Geometry check sheet. Reference: the model listing, model coordinates, mm. A direction names the side the tool comes from. Coordinates: 2 decimals unless noted, no trailing zeros. Order: outer loops, then holes, each group sorted by start corner. A loop starts at its lowest first (then second) coordinate and runs counter-clockwise, first axis right, second up. Notation, with made-up numbers: (26.25, 65) - (66.25, 65) arc R15 ccw to (66.25, 73) - close; hole circle Ø7 at (37.5, 6.25). An arc over 180 degrees is marked (long way). One line per item, written item: value. Start each with the question number.
Autodesk Inventor part; units mm, degrees
ref_plane "YZ Plane" through (0, 0, 0) normal (1, 0, 0) x (0, 1, 0)
ref_plane "XZ Plane" through (0, 0, 0) normal (0, 1, 0) x (-1, 0, 0)
ref_plane "XY Plane" through (0, 0, 0) normal (0, 0, 1) x (1, 0, 0)
sketch "Sketch1" plane through (0, 0, 0) normal (0, 0, 1) x (1, 0, 0)
  line L0 (-64, 10) -> (0, 10)
  line L1 (0, 10) -> (0, 0)
  line L2 (0, 0) -> (-64, 0)
  line L3 (-64, 0) -> (-64, 10)
  dimension "d0" = 64
  dimension "d1" = 10
extrude "Extrusion1" add sketch "Sketch1" along normal blind 50
sketch "Sketch2" plane through (0, 0, 50) normal (0, 0, 1) x (1, 0, 0)
  line L0 (0, 10) -> (-64, 10)
  line L1 (-64, 10) -> (-64, 0)
  line L2 (-64, 0) -> (0, 0)
  line L3 (0, 0) -> (0, 10)
  circle A0 centre (-57, 5) radius 2.5
  circle A1 centre (-7, 5) radius 2.5
  line L4 (-32, 17) -> (-32, -12)
  line L5 (-64, 10) -> (-64, 0)
  line L6 (-64, 5) -> (0, 5)
  dimension "d4" = 50
  dimension "d5" = 5
  dimension "d6" = 32
extrude "Extrusion2" cut sketch "Sketch2" against normal blind 18 contours L6 A1 | A1 L6 | L6 A0 | A0 L6
sketch "Sketch3" plane through (0, 0, 50) normal (0, 0, 1) x (1, 0, 0)
  circle A0 centre (-7, 5) radius 2.5
  circle A1 centre (-57, 5) radius 2.5
  line L0 (0, 10) -> (-64, 10)
  line L1 (-64, 10) -> (-64, 0)
  line L2 (-64, 0) -> (0, 0)
  line L3 (0, 0) -> (0, 10)
  line L4 (-64, 0) -> (0, 0)
  line L5 (-50, 10) -> (-14, 10)
  line L6 (-14, 10) -> (-14, 0)
  line L7 (-14, 0) -> (-50, 0)
  line L8 (-50, 0) -> (-50, 10)
  dimension "d9" = 14
  dimension "d10" = 14
ref_plane "Work Plane1" through (-32, 0, 0) normal (-1, 0, 0) x (0, 0, 1)
extrude "Extrusion3" cut sketch "Sketch3" against normal blind 15 contours L6 L2 L8 L0
sketch "Sketch4" plane through (-64, 0, 0) normal (0, -1, 0) x (1, 0, 0)
  line L0 (14, 35) -> (14, 50)
  line L1 (0, 50) -> (14, 50)
  line L2 (0, 0) -> (0, 50)
  line L3 (64, 0) -> (0, 0)
  line L4 (64, 0) -> (64, 50)
  line L5 (50, 50) -> (64, 50)
  line L6 (50, 50) -> (50, 35)
  line L7 (50, 35) -> (14, 35)
  line L8 (9.5, 50) -> (9.5, 32)
  line L9 (4.5, 50) -> (4.5, 32)
sketch "Sketch5" plane through (-64, 0, 0) normal (0, -1, 0) x (1, 0, 0)
  line L0 (4, 45) -> (10, 45)
  line L1 (10, 45) -> (10, 42)
  line L2 (10, 42) -> (4, 42)
  line L3 (4, 42) -> (4, 45)
  line L4 (4.5, 50) -> (9.5, 50)
  line L5 (7, 50) -> (7, 38)
  line L6 (0, 50) -> (14, 50)
  point P0 (64, 0)
  point P1 (7, 50)
  dimension "d13" = 6
  dimension "d14" = 3
  dimension "d15" = 5
extrude "Extrusion4" cut sketch "Sketch5" against normal blind 8.5
mirror "Mirror1" about plane through (-32, 0, 0) normal (-1, 0, 0) of "Extrusion4"
sketch "Sketch6" plane through (0, 0, 0) normal (0, 0, -1) x (-1, 0, 0)
  line L0 (64, 10) -> (0, 10)
  line L1 (0, 10) -> (0, 0)
  line L2 (0, 0) -> (64, 0)
  line L3 (64, 0) -> (64, 10)
  line L4 (0, 0) -> (64, 0)
  line L5 (64, 0) -> (64, -15)
  line L6 (64, -15) -> (0, -15)
  line L7 (0, -15) -> (0, 0)
  dimension "d30" = 15
extrude "Extrusion5" add sketch "Sketch6" against normal blind 4 contours L5 L6 L7 L2
sketch "Sketch7" plane through (0, 0, 4) normal (0, 0, 1) x (1, 0, 0)
  line L0 (0, -15) -> (0, 0)
  line L1 (-64, 0) -> (0, 0)
  line L2 (-64, 0) -> (-64, -15)
  line L3 (-64, -15) -> (0, -15)
  line L4 (-54, -7) -> (-10, -7) construction
  line L5 (-54, -9.5) -> (-10, -9.5)
  line L6 (-10, -4.5) -> (-54, -4.5)
  arc A0 (-54, -4.5) -> (-54, -9.5) centre (-54, -7) ccw
  arc A1 (-10, -9.5) -> (-10, -4.5) centre (-10, -7) ccw
  point P0 (-32, -7)
  dimension "d20" = 5
  dimension "d22" = 10
  dimension "d23" = 10
  dimension "d24" = 7
extrude "Extrusion6" cut sketch "Sketch7" against normal through all contours A0 L6 A1 L5
chamfer "Chamfer1" distance 1 angle 45 4 edges at (-32, -4.5, 4) (-7.5, -7, 4) (-32, -9.5, 4) (-56.5, -7, 4)
fillet "Fillet1" radius 2 26 edges at (-64, 10, 25) (-50, 10, 42.5) (-57, 10, 50) (-50, 5, 50) (-64, 5, 50) (-64, 0, 27) (-32, 10, 35) (-14, 10, 42.5) (-14, 5, 50) (-7, 10, 50) (0, 5, 50) (0, 10, 25) (-14, 5, 35) (-32, 0, 35) (-50, 5, 35) (-57, 0, 50) (-50, 0, 42.5) (-14, 0, 42.5) (-32, 0, 4) (0, -7.5, 4) (-32, -15, 4) (-64, -7.5, 4) (-64, -15, 2) (0, -15, 2) (-7, 0, 50) (0, 0, 27)
properties part number "soporte0.2"
Q1. Gauge pin test, flat ends, axial feed: P1, Ø3.5, axis at y = 4.5, z = 44, coming from the +X side; P2, Ø5.5, axis at x = -26, y = -6, coming from the +Z side; P3, Ø1, axis at x = -18.5, z = 31.5, coming from the -Y side; P4, Ø3, axis at x = -33, y = 4, coming from the +Z side. Record the tip position at first contact, or that the pin passes through.
Q2. Release check for a two-part mould opening along X. For faces 1 (the cylindrical face through (-7.07, 0.57, 49.4)), 2 (the cylindrical face through (-63.4, 9.43, 24.34)), 3 (the flat face through (-7, 8.5, 44)) record: released by +X, released by -X, zero draft, split by the parting line, or undercut.
Q3. Set-up check for faces 4 (the cylindrical face through (-63.43, 0.6, 27.29)), 5 (the flat face through (-7, 5, 32)), 6 (the flat face through (-50, 5, 43)): record each of +Z, -Z, +X, -X, +Y, -Y from which the full face is reachable in a straight line by a thin tool's end or side.
Q4. Material ranges on probe 1 along X at (y, z) = (5, 47); probe 2 along Y at (x, z) = (-7, 40); probe 3 along Y at (x, z) = (-58, 44.5), recorded low to high.
Q5. Cross-section at B-B, the plane y = -7. Enter the section's corners in (x, z).
Q6. Cross-section at C-C, the plane z = 16. Enter the section's corners in (x, y).
Q7. Cross-section at A-A, the plane x = -31. Enter the section's corners in (y, z), and give its area (3 significant figures).
Check result:
1. P1: stops at x = 0
1. P2: stops at z = 4
1. P3: stops at y = 0
1. P4: stops at z = 35
2. face 1: zero draft
2. face 2: released by -X
2. face 3: undercut
3. face 4: +Z, -X, -Y
3. face 5: +Z
3. face 6: +Z, +Y, -Y
4. probe 1: x = -64 to -59.5, -54.5 to -50, -14 to -9.5, -4.5 to 0
4. probe 2: y = 0 to 2.5, 7.5 to 10
4. probe 3: y = 8.5 to 10
5. outline: (-64, 0) - (-56.5, 0) - (-56.5, 3) - (-57.5, 4) - (-62, 4) arc R2 ccw to (-64, 2) - close; (-7.5, 0) - (0, 0) - (0, 2) arc R2 ccw to (-2, 4) - (-6.5, 4) - (-7.5, 3) - close
6. outline: (-64, 2) arc R2 ccw to (-62, 0) - (-2, 0) arc R2 ccw to (0, 2) - (0, 8) arc R2 ccw to (-2, 10) - (-62, 10) arc R2 ccw to (-64, 8) - close
7. outline: (-15, 0) - (-9.5, 0) - (-9.5, 3) - (-10.5, 4) - (-13, 4) arc R2 ccw to (-15, 2) - close; (-4.5, 0) - (10, 0) - (10, 33) arc R2 ccw to (8, 35) - (2, 35) arc R2 ccw to (0, 33) - (0, 6) arc R2 cw to (-2, 4) - (-3.5, 4) - (-4.5, 3) - close
7. area: 387 mm2
